Study the drawing (mm; zero at the part's minimum x, y, z) and answer. Coordinates: 2 decimals unless noted, no trailing zeros. Order: outer loops, then holes, each group sorted by start corner. A loop starts at its lowest first (then second) coordinate and runs counter-clockwise, first axis right, second up. Notation, with made-up numbers: (47.5, 65) -> (93.5, 65) arc R30 ccw to (93.5, 100) -> close; hole circle Ø8 at (4.25, -24.5). An arc over 180 degrees is marked (long way). Answer as CSV lines item,"result". Start each with the question number.
Item 1: Section A-A (x = 26) is taken. Write down the section's boundary in (y, z), then the cut area to 3 significant figures.
Item 2: Straight lines are drawn through the part: L1, parallel to Y at x = 26, z = 0.6; L2, parallel to Y at x = 28.5, z = 0.2; L3, parallel to X at y = 17.5, z = 0.2. For each, find the intervals that lie inside material, in ascending order.
Item 3: Section B-B (y = 15.9) is taken. Write down the section's boundary in (x, z), then the cut area to 3 significant figures.
Item 4: Section C-C (z = 2.55) is taken. Write down the section's boundary in (x, y), then the cut area to 3 significant figures.
Item 5: This flat-tipped pin is pushed along its axis until it touches: pin 1 Ø6 at (x, y) = (14, 17) entering from -Z. Where does it stop, or does it pass through?
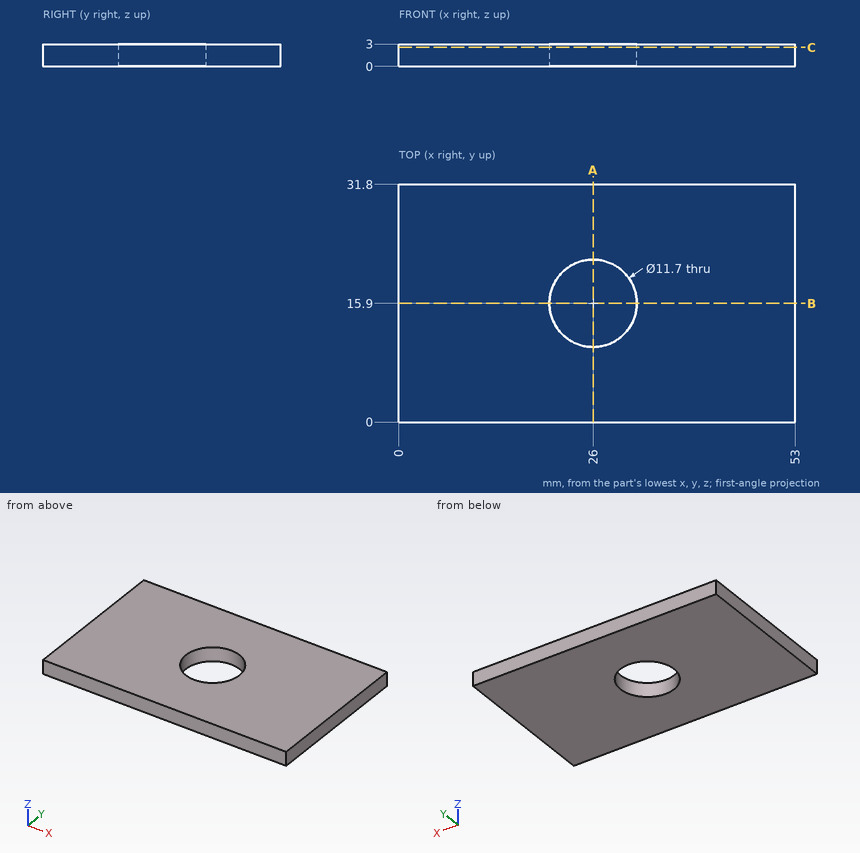
Checked values:
1,outline,"(0, 0) -> (10.05, 0) -> (10.05, 3) -> (0, 3) -> close; (21.75, 0) -> (31.8, 0) -> (31.8, 3) -> (21.75, 3) -> close"
1,area,"60.3 mm^2"
2,L1,"y = 0 to 10.05, 21.75 to 31.8"
2,L2,"y = 0 to 10.61, 21.19 to 31.8"
2,L3,"x = 0 to 20.37, 31.63 to 53"
3,outline,"(0, 0) -> (20.15, 0) -> (20.15, 3) -> (0, 3) -> close; (31.85, 0) -> (53, 0) -> (53, 3) -> (31.85, 3) -> close"
3,area,"124 mm^2"
4,outline,"(0, 0) -> (53, 0) -> (53, 31.8) -> (0, 31.8) -> close; hole circle Ø11.7 at (26, 15.9)"
4,area,"1,580 mm^2"
5,pin 1,"stops at z = 0"
